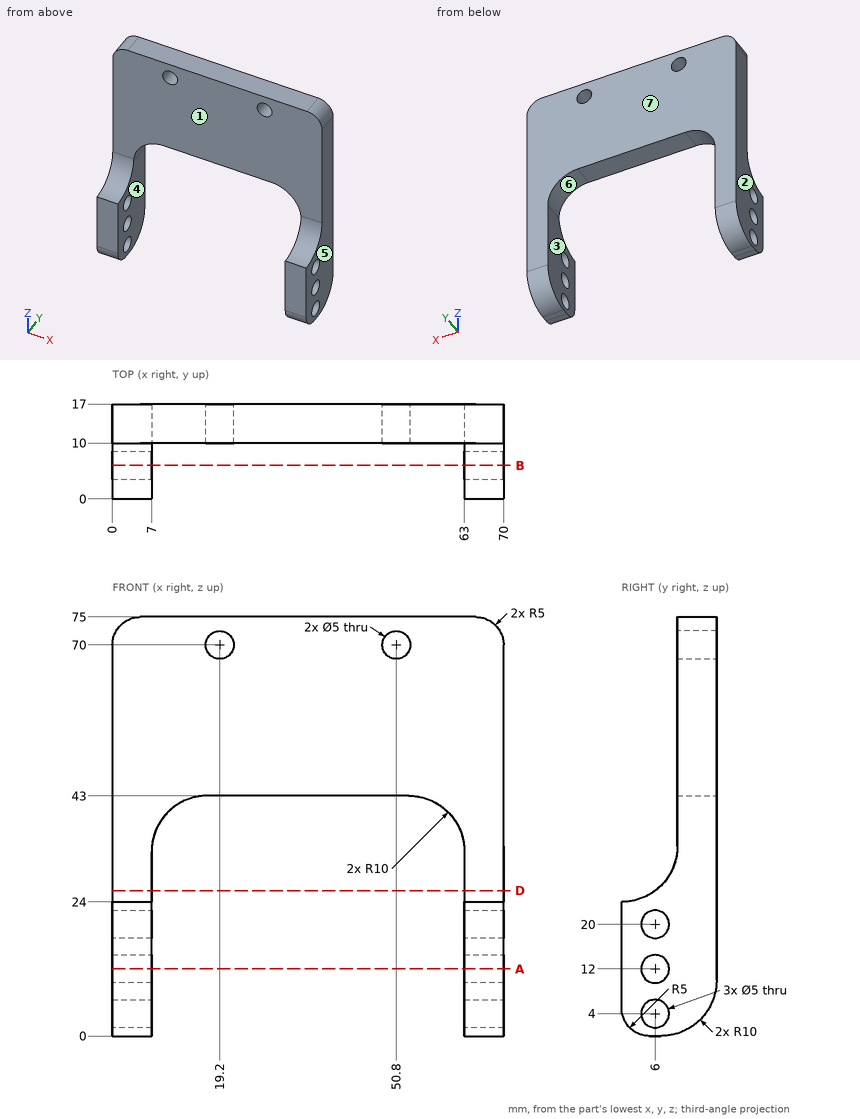
Geometry: see drawing. Coordinates: mm, zero at the bounding-box minimum. A direction names the side the tool comes from. Coordinates: 2 decimals unless noted, no trailing zeros. Loops run counter-clockwise (first coordinate to the right, second up) from the corner with the lowest first, then second, coordinate; pieces in that order, holes last. Notation, with made-up numbers: M -35.75,82 L 14.25,82 A21 ccw 14.25,110 Z; hole C 4,-25 d10. An arc over 180 degrees is marked long. Answer in a Markdown table with one row per item.
1. Section B-B, the plane y = 6. Count the separate pieces of the cut face and the enclosed holes in it, then the cut area to 3 significant figures.
Response:
| item | result |
|---|---|
| separate pieces | 8 |
| enclosed holes | 0 |
| area | 154 mm2 |
2. Material intervals for line 1 (X direction, y = 11.5, z = 70); line 2 (Y direction, x = 65, z = 20); line 3 (X direction, y = 13.25, z = 5.5), sorted ascending.
Response:
| item | result |
|---|---|
| line 1 | x = 0 to 16.7, 21.7 to 48.3, 53.3 to 70 |
| line 2 | y = 0 to 3.5, 8.5 to 17 |
| line 3 | x = 0 to 7, 63 to 70 |
3. Section D-D, the plane z = 26. Output: boundary loops of the cut face in (x, y), then the cut area to 3 significant figures.
Response:
| item | result |
|---|---|
| outline | M 0,6 L 7,6 L 7,17 L 0,17 Z; M 63,6 L 70,6 L 70,17 L 63,17 Z |
| area | 154 mm2 |
4. Section A-A, the plane z = 12. Output: boundary loops of the cut face in (x, y), then the cut area to 3 significant figures.
Response:
| item | result |
|---|---|
| outline | M 0,0 L 7,0 L 7,3.5 L 0,3.5 Z; M 0,8.5 L 7,8.5 L 7,17 L 0,17 Z; M 63,0 L 70,0 L 70,3.5 L 63,3.5 Z; M 63,8.5 L 70,8.5 L 70,17 L 63,17 Z |
| area | 168 mm2 |
5. First-contact query: pin 1 (1 mm diameter, centred on x = 22.5, z = 61.5, fed in from -Y); pin 2 (3.5 mm diameter, centred on x = 41.5, y = 14, fed in from -Z). Flat tips, straight axial feed; report the tip coordinate or a pass-through.
Response:
| item | result |
|---|---|
| pin 1 | stops at y = 10 |
| pin 2 | stops at z = 43 |
6. Draft query along X for the marked faces 4, 5, 6 and 7. Return one class per face: pulls with the +X half, pulls with the -X half, needs draft (parallel to the pull), parting line crosses it, or undercut.
Response:
| item | result |
|---|---|
| face 4 | undercut |
| face 5 | pulls with the +X half |
| face 6 | undercut |
| face 7 | needs draft |
7. Reachability of the marked faces 1, 2 and 3 from +Z, -Z, +X, -X, +Y, -Y: full face, straight path, thin tool, end or side. Return the list, or none.
Response:
| item | result |
|---|---|
| face 1 | +Z, +X, -X, -Y |
| face 2 | +Z, -Z, -X, +Y, -Y |
| face 3 | -Z, +Y, -Y |
